Part model, mm, in its own coordinate system. A direction names the side the tool comes from. Round coordinates to 2 decimals unless told otherwise and drop trailing zeros. Loops run counter-clockwise (first coordinate to the right, second up) from the corner with the lowest first, then second, coordinate; pieces in that order, holes last. Notation, with made-up numbers: M 19,-39.5 L 42,-39.5 A10 ccw 42,-23.5 Z; hole C 73.5,3 d2. An arc over 180 degrees is marked long. Put each result on its own line as item: value. Start each with the question number.
1) Pull direction X, two halves, no side cores. Call faces 1 (the cylindrical face through (-8.523, -2.904, 6.439)), 2 (the cylindrical face through (-49.127, -12.467, 6.439)), 3 (the flat face through (-64.6, -6.9, 38.1)): +X half, -X half, draft (parallel to the pull), parting line (faces both ways), or undercut.
2) Slice it at A-A on x = -41. Give the cut face in (y, z).
3) Which spindle directions (+Z, -Z, +X, -X, +Y, -Y) get a long thin tool onto all of the face, cutting with end or side? Do faces 4 (the flat face through (-42, 0, 6)), 5 (the flat face through (-30, -18.957, 6)). Say none if no direction does.
4) Slice it at D-D on z = 26.5. Give the cut face in (x, y).
5) Slice it at C-C on z = 8. Give the cut face in (x, y).
6) Drop flat-ended pins along their axis: pin 1 Ø12.5 at (x, y) = (-37, -18.5) entering from +Z; pin 2 Ø2 at (y, z) = (-17, 20.5) entering from -X; pin 3 Ø8 at (x, z) = (-53, 28.5) entering from -Y. Give the stop position or say it passes through.
7) Probe line 1 along X through (y, z) = (-15.5, 7); line 2 along X through (y, z) = (-8.25, 3.5); line 3 along Y through (x, z) = (-68, 27.5). List the from-to ranges inside material, lowest first.
8) Slice it at B-B on y = -8.25. Give the cut face in (x, z).
```python
from build123d import *

# Parameters (mm, degrees)
F1_DEPTH = 25.4
F3_DEPTH = 12.701
F4_R     = 6.35
F5_DEPTH = 38.101
F7_DEPTH = 25.4


with BuildPart() as f1:
    # F0 (on Front) → F1 (new body)
    with BuildSketch(Plane.XZ):
        Polygon((-54.9375581781, 38.1), (-80.3375581781, 38.1), (-80.3375581781, 0), (-4.1375581781, 0), (-4.1375581781, 12.7), (-54.9375581781, 12.7), align=None)
    extrude(amount=F1_DEPTH)

    # F2 (on face) → F3 (cut, through all)
    with BuildSketch(Plane.XY.offset(12.7)):
        with BuildLine():
            ThreePointArc((-36.4283830897, -12.6069579273), (-38.2882550292, -8.1168298668), (-42.7783830897, -6.2569579273))
            ThreePointArc((-42.7783830897, -6.2569579273), (-49.1283830897, -12.6069579273), (-42.7783830897, -18.9569579273))
            ThreePointArc((-42.7783830897, -18.9569579273), (-38.2882550292, -17.0970859879), (-36.4283830897, -12.6069579273))
        make_face()
        with BuildLine():
            ThreePointArc((-16.3607828855, -18.9569579273), (-22.7107828855, -12.6069579273), (-16.3607828855, -6.2569579273))
            Line((-16.3607828855, -6.2569579273), (-42.7783830897, -6.2569579273))
            ThreePointArc((-42.7783830897, -6.2569579273), (-38.2882550292, -8.1168298668), (-36.4283830897, -12.6069579273))
            ThreePointArc((-36.4283830897, -12.6069579273), (-38.2882550292, -17.0970859879), (-42.7783830897, -18.9569579273))
            Line((-42.7783830897, -18.9569579273), (-16.3607828855, -18.9569579273))
        make_face()
        with BuildLine():
            ThreePointArc((-16.3607828855, -18.9569579273), (-11.870654825, -17.0970859879), (-10.0107828855, -12.6069579273))
            ThreePointArc((-10.0107828855, -12.6069579273), (-11.870654825, -8.1168298668), (-16.3607828855, -6.2569579273))
            ThreePointArc((-16.3607828855, -6.2569579273), (-22.7107828855, -12.6069579273), (-16.3607828855, -18.9569579273))
        make_face()
        with BuildLine():
            ThreePointArc((-16.3607828855, 0), (-8.4297023381, -2.981044621), (-4.1375581781, -10.2862594838))
            Line((-4.1375581781, -10.2862594838), (-4.1375581781, 0))
            Line((-4.1375581781, 0), (-16.3607828855, 0))
        make_face()
        with BuildLine():
            ThreePointArc((-4.1375581781, -15.1137405162), (-8.4297023381, -22.418955379), (-16.3607828855, -25.4))
            Line((-16.3607828855, -25.4), (-4.1375581781, -25.4))
            Line((-4.1375581781, -25.4), (-4.1375581781, -15.1137405162))
        make_face()
    extrude(amount=-F3_DEPTH, mode=Mode.SUBTRACT)

    # F4 (on face) → F5 (cut, through all)
    with BuildSketch(Plane.XY.offset(38.1)):
        with BuildLine():
            ThreePointArc((-80.3375581781, -12.7), (-76.6178142992, -3.7197438789), (-67.6375581781, 0))
            Line((-67.6375581781, 0), (-80.3375581781, 0))
            Line((-80.3375581781, 0), (-80.3375581781, -12.7))
        make_face()
        with BuildLine():
            Line((-80.3375581781, -25.4), (-67.6375581781, -25.4))
            ThreePointArc((-67.6375581781, -25.4), (-76.6178142992, -21.6802561211), (-80.3375581781, -12.7))
            Line((-80.3375581781, -12.7), (-80.3375581781, -25.4))
        make_face()
        with Locations((-67.6375581781, -12.7)):
            Circle(F4_R)
    extrude(amount=-F5_DEPTH, mode=Mode.SUBTRACT)

    # F6 (on face) → F7 (cut)
    with BuildSketch(Plane.XY.offset(38.1)):
        with BuildLine():
            ThreePointArc((-54.9375581781, -12.7), (-58.657302057, -21.6802561211), (-67.6375581781, -25.4))
            Line((-67.6375581781, -25.4), (-54.9375581781, -25.4))
            Line((-54.9375581781, -25.4), (-54.9375581781, -12.7))
        make_face()
        with BuildLine():
            ThreePointArc((-67.6375581781, 0), (-58.657302057, -3.7197438789), (-54.9375581781, -12.7))
            Line((-54.9375581781, -12.7), (-54.9375581781, 0))
            Line((-54.9375581781, 0), (-67.6375581781, 0))
        make_face()
    extrude(amount=-F7_DEPTH, mode=Mode.SUBTRACT)


solid = f1.part
```
Recorded:
1. face 1: +X half
1. face 2: undercut
1. face 3: draft
2. outline: M -25.4,0 L -18.96,0 L -18.96,12.7 L -25.4,12.7 Z; M -6.26,0 L 0,0 L 0,12.7 L -6.26,12.7 Z
3. face 4: +Z, -Z, +X, -X, +Y
3. face 5: +Z, -Z
4. outline: C -67.64,-12.7 d25.4; hole C -67.64,-12.7 d12.7
5. outline: M -67.64,-25.4 L -16.36,-25.4 A12.7 ccw -4.14,-15.11 L -4.14,-10.29 A12.7 ccw -16.36,0 L -67.64,0 A12.7 ccw Z; hole C -67.64,-12.7 d12.7; hole M -42.78,-18.96 L -16.36,-18.96 A6.35 ccw -16.36,-6.26 L -42.78,-6.26 A6.35 ccw Z
6. pin 1: stops at z = 12.7
6. pin 2: stops at x = -79.9
6. pin 3: stops at y = -19.64
7. line 1: x = -80.03 to -73.34, -61.94 to -48.43, -10.71 to -4.22
7. line 2: x = -79.53 to -72.17, -63.11 to -47.4, -11.74 to -4.71
7. line 3: y = -25.39 to -19.04, -6.36 to -0.01
8. outline: M -79.53,0 L -72.17,0 L -72.17,38.1 L -79.53,38.1 Z; M -63.11,0 L -47.4,0 L -47.4,12.7 L -55.74,12.7 L -55.74,38.1 L -63.11,38.1 Z; M -11.74,0 L -4.71,0 L -4.71,12.7 L -11.74,12.7 Z
